Part model, mm, in its own coordinate system. A direction names the side the tool comes from. Coordinates: 2 decimals unless noted, no trailing zeros. Use a Markdown table: item, result.
```python
from build123d import *

# Parameters (mm, degrees)
CHAMFER_963_SIZE             = 1
SKETCH_2_W                   = 4.1
SKETCH_2_H                   = 2.45
PATTERN_LINEAR_O_2_COUNT     = 2
PATTERN_LINEAR_O_2_PITCH     = 9
PATTERN_CIRCULAR_M10_COUNT   = 8
PATTERN_CIRCULAR_M10_2_COUNT = 3


# Read off the part's stored shape, not the designer's step: トレイ支柱 M4（内側）
with BuildPart() as part:
    # ｽｹｯﾁ1 → Revolve 926 (revolve)
    with BuildSketch(Plane.XY, mode=Mode.PRIVATE) as revolve_926_sk:
        Polygon((-12, 0), (-12, 79), (0, 79), (0, 70.95), (25, 70.95), (25, 62), (0, 62), (0, 0), align=None)
    revolve(revolve_926_sk.sketch.rotate(Axis((0, 0, 0), (1, 0, 0)), 90), axis=Axis((0, 0, 0), (1, 0, 0)))

    # Chamfer 963
    chamfer_963_edges = [part.edges().sort_by_distance(p)[0] for p in [
        (25, 0, -70.95),
    ]]
    chamfer(chamfer_963_edges, length=CHAMFER_963_SIZE)

    # ｽｹｯﾁ2 → Oリング溝入れ G-135 (revolve, cut)
    with BuildSketch(Plane.XY, mode=Mode.PRIVATE) as o_g_135_sk:
        with Locations((7.05, 69.725)):
            Rectangle(SKETCH_2_W, SKETCH_2_H)
    o_g_135 = revolve(o_g_135_sk.sketch.rotate(Axis((0, 0, 0), (1, 0, 0)), 90), axis=Axis((0, 0, 0), (1, 0, 0)), mode=Mode.SUBTRACT)

    # Oリング溝 2 本目: Oリング溝入れ G-135 ×2
    with Locations(*[(i * PATTERN_LINEAR_O_2_PITCH, 0, 0) for i in range(1, PATTERN_LINEAR_O_2_COUNT)]):
        add(o_g_135, mode=Mode.SUBTRACT)

    # ｽｹｯﾁ3 → Hole Wizard M10 (revolve, cut)
    with BuildSketch(Plane(origin=(-12, 45, 0), x_dir=(0, 0, 1), z_dir=(0, 1, 0))):
        Polygon((0, 0), (0, 15.553657631), (4.25, 13), (4.25, 0), align=None)
    hole_wizard_m10 = revolve(axis=Axis((-18.35, 45, 0), (1, 0, 0)), mode=Mode.SUBTRACT)

    # Pattern Circular M10: Hole Wizard M10 ×8 about axis
    pattern_circular_m10_axis = Axis((0, 0, 0), (1, 0, 0))
    for i in range(1, PATTERN_CIRCULAR_M10_COUNT):
        add(hole_wizard_m10.rotate(pattern_circular_m10_axis, i * 360 / PATTERN_CIRCULAR_M10_COUNT), mode=Mode.SUBTRACT)

    # ｽｹｯﾁ5 → Hole Wizard M10 2 (revolve, cut)
    with BuildSketch(Plane(origin=(-12, 15, 0), x_dir=(0, 0, 1), z_dir=(0, 1, 0))):
        Polygon((0, 0), (0, 15.553657631), (4.25, 13), (4.25, 0), align=None)
    hole_wizard_m10_2 = revolve(axis=Axis((-18.35, 15, 0), (1, 0, 0)), mode=Mode.SUBTRACT)

    # Pattern Circular M10 2: Hole Wizard M10 2 ×3 about axis
    pattern_circular_m10_2_axis = Axis((0, 0, 0), (1, 0, 0))
    for i in range(1, PATTERN_CIRCULAR_M10_2_COUNT):
        add(hole_wizard_m10_2.rotate(pattern_circular_m10_2_axis, i * 360 / PATTERN_CIRCULAR_M10_2_COUNT), mode=Mode.SUBTRACT)

    # トレイ支柱 M4（内側） outline → トレイ支柱 M4（内側） (revolve, cut)
    with BuildSketch(Plane(origin=(0, -45, 22), x_dir=(0, 1, 0), z_dir=(0, 0, -1))):
        Polygon((0, 0), (0, -8.991420021), (1.65, -8), (1.65, 0), align=None)
    hole_wizard_m4 = revolve(axis=Axis((0, -45, 22), (1, 0, 0)), mode=Mode.SUBTRACT)

    # トレイ支柱 M4（内側・対称）: トレイ支柱 M4（内側） across plane
    add(hole_wizard_m4.mirror(Plane.XY), mode=Mode.SUBTRACT)


solid = part.part
```
Item 1: Drill centre lines: probe 1 along Z at (x, y) = (-6, -45); probe 2 along X at (y, z) = (64, 29.5); probe 3 along X at (y, z) = (-15, 46). Where is each one in solid material? Low to high.
From the geometry:
| item | result |
|---|---|
| probe 1 | -64.93 to -23.65, -20.35 to -4.25, 4.25 to 20.35, 23.65 to 64.93 |
| probe 2 | -12 to 5, 9.1 to 14, 18.1 to 24.48 |
| probe 3 | -12 to 0 |
Item 2: Which spindle directions (+Z, -Z, +X, -X, +Y, -Y) get a long thin tool onto all of the face, cutting with end or side? Do faces 1 (the face through (21.091, -47.951, -52.293)), 2 (the face through (9.1, -58, 37)), 3 (the face through (-6.084, -35.747, 30.195)). Say none if no direction does.
From the geometry:
| item | result |
|---|---|
| face 1 | +X |
| face 2 | none |
| face 3 | +X, -X |
Item 3: Two-plate mould, pull along X, no slides. Class faces 4 (the face through (-6.08, 3.37, 47.59)), 5 (the face through (14, -58, 37)), 6 (the face through (0, -30, -65)): pulls with the +X half, pulls with the -X half, needs draft (parallel to the pull), parting line crosses it, or undercut.
From the geometry:
| item | result |
|---|---|
| face 4 | needs draft |
| face 5 | undercut |
| face 6 | pulls with the +X half |
Item 4: Drop flat-ended pins along their axis: P1, Ø11, axis at y = -7.5, z = -12.99, coming from the +X side; P2, Ø5, axis at x = 13.5, z = -12, coming from the +Y side; P3, Ø12, axis at x = 11, z = 4.5, coming from the +Y side. Give the stop position or say it passes through.
From the geometry:
| item | result |
|---|---|
| P1 | x = 0 |
| P2 | y = 70.31 |
| P3 | y = 70.95 |
Item 5: Band-saw the part on A-A, the plane x = -5.5. Count the separate pieces of the cut face and the enclosed holes in it, then the cut area to 3 significant figures.
From the geometry:
| item | result |
|---|---|
| separate pieces | 1 |
| enclosed holes | 13 |
| area | 19,000 mm^2 |
